Geometry: see drawing. Coordinates: mm, zero at the bounding-box minimum. Give positions to 0.01 mm unless a question says otherwise; leave off trailing zeros. Write each loop counter-clockwise with the first axis right and the second up, starting at its lowest first coordinate (ties: lowest second). Pieces come first, ordered by that corner, then holes. Notation, with made-up numbers: M -24,86 L 24,86 A26 cw 24,102 Z; hole C 52,75 d3. An arc over 180 degrees is marked long. Use one line per item in the form item = value. Start each with the question number.
Item 1: Material intervals for line 1 along X through (y, z) = (113.5, 2.4); line 2 along X through (y, z) = (63, 1.7); line 3 along Y through (x, z) = (70, 1.65), sorted ascending. Write a range as from..to.
Item 2: Section query D-D on y = 59.25. Return loops of the section in (x, z), then the cut area to 3 significant figures.
Item 3: Section query B-B on y = 113.5. Return loops of the section in (x, z), then the cut area to 3 significant figures.
Item 4: Section query A-A on x = 10. Return loops of the section in (y, z), then the cut area to 3 significant figures.
Item 5: Section query C-C on x = 40. Return loops of the section in (y, z), then the cut area to 4 significant figures.
Item 6: Contact query for a flat-ended pin moving along its axis: P1, Ø2.5, axis at x = 70, y = 5, coming from the -Z side. Output: stop coordinate, or through.
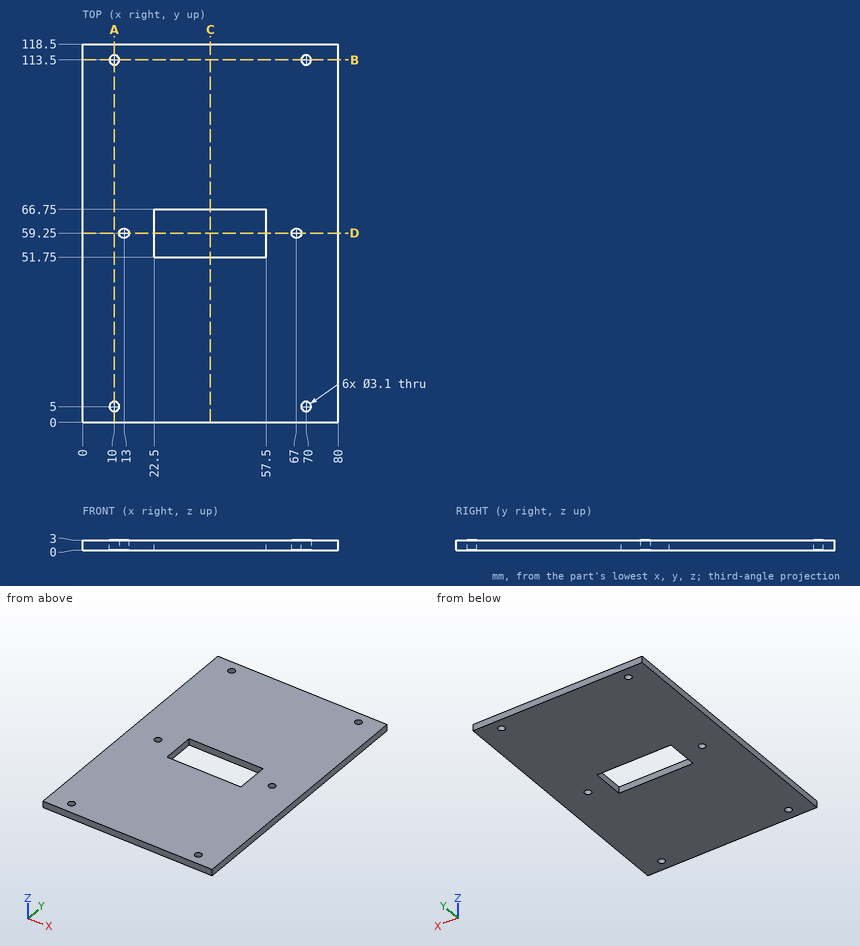
Answer sheet:
q1.line_1 = 0..8.45, 11.55..68.45, 71.55..80
q1.line_2 = 0..22.5, 57.5..80
q1.line_3 = 0..3.45, 6.55..111.95, 115.05..118.5
q2.outline = M 0,0 L 11.45,0 L 11.45,3 L 0,3 Z; M 14.55,0 L 22.5,0 L 22.5,3 L 14.55,3 Z; M 57.5,0 L 65.45,0 L 65.45,3 L 57.5,3 Z; M 68.55,0 L 80,0 L 80,3 L 68.55,3 Z
q2.area = 116 mm2
q3.outline = M 0,0 L 8.45,0 L 8.45,3 L 0,3 Z; M 11.55,0 L 68.45,0 L 68.45,3 L 11.55,3 Z; M 71.55,0 L 80,0 L 80,3 L 71.55,3 Z
q3.area = 221 mm2
q4.outline = M 0,0 L 3.45,0 L 3.45,3 L 0,3 Z; M 6.55,0 L 111.95,0 L 111.95,3 L 6.55,3 Z; M 115.05,0 L 118.5,0 L 118.5,3 L 115.05,3 Z
q4.area = 337 mm2
q5.outline = M 0,0 L 51.75,0 L 51.75,3 L 0,3 Z; M 66.75,0 L 118.5,0 L 118.5,3 L 66.75,3 Z
q5.area = 310.5 mm2
q6.P1 = through
